Check sheet for the modelled part. Datum: model origin and axes. Units: mm. Face numbers are marked on the shaded views. A direction names the side the tool comes from. Round coordinates to 2 decimals unless told otherwise and drop trailing zeros. Loops run counter-clockwise (first coordinate to the right, second up) from the corner with the lowest first, then second, coordinate; pieces in that order, holes last. Notation, with made-up numbers: (78.5, -31) - (86.5, -31) arc R9 ccw to (86.5, -23) - close; hole circle Ø7 at (18.5, 58.5). An arc over 180 degrees is marked (long way). Put each result on its own line as item: value.
```python
from build123d import *

# Parameters (mm, degrees)
EXTRUDE_1_DEPTH = 6
EXTRUDE_2_DEPTH = 7
SKETCH_2_6_W    = 17.5
SKETCH_2_6_H    = 7
EXTRUDE_3_DEPTH = 28.5
CHAMFER_1_SIZE  = 4
HOLE_WIZARD_1_D = 8
FILLET_1_R      = 1
CHAMFER_2_SIZE  = 1


with BuildPart() as part:
    # Sketch 2 → Extrude 1 (new, symmetric)
    with BuildSketch(Plane.XY):
        with BuildLine():
            Line((-22.5, 0), (0, 0))
            Line((0, 0), (0, 20))
            Line((0, 20), (-10.5, 20))
            ThreePointArc((-10.5, 20), (-12, 21.5), (-10.5, 23))
            Line((-10.5, 23), (-10.5, 45))
            ThreePointArc((-10.5, 45), (-12, 46.5), (-10.5, 48))
            Line((-10.5, 48), (0, 48))
            Line((0, 48), (0, 55))
            Line((0, 55), (-22.5, 55))
            Line((-22.5, 55), (-22.5, 0))
        make_face()
        with BuildLine():
            Line((0, 20), (0, 0))
            Line((0, 0), (22.5, 0))
            Line((22.5, 0), (22.5, 55))
            Line((22.5, 55), (0, 55))
            Line((0, 55), (0, 48))
            Line((0, 48), (10.5, 48))
            ThreePointArc((10.5, 48), (11.560660172, 47.560660172), (12, 46.5))
            ThreePointArc((12, 46.5), (11.560660172, 45.439339828), (10.5, 45))
            Line((10.5, 45), (10.5, 23))
            ThreePointArc((10.5, 23), (11.560660172, 22.560660172), (12, 21.5))
            ThreePointArc((12, 21.5), (11.560660172, 20.439339828), (10.5, 20))
            Line((10.5, 20), (0, 20))
        make_face()
    extrude(amount=EXTRUDE_1_DEPTH, both=True)

    # Sketch 2_5 → Extrude 2 (add, symmetric)
    with BuildSketch(Plane.XY):
        Polygon((-22.5, 69), (-22.5, 55), (0, 55), (0, 62), (-17.5, 62), (-17.5, 69), align=None)
        Polygon((0, 55), (22.5, 55), (22.5, 69), (17.5, 69), (17.5, 62), (0, 62), align=None)
    extrude(amount=EXTRUDE_2_DEPTH, both=True)

    # Sketch 2_6 → Extrude 3 (add, symmetric)
    with BuildSketch(Plane.XY):
        with Locations((-8.75, 65.5)):
            Rectangle(SKETCH_2_6_W, SKETCH_2_6_H)
        with Locations((8.75, 65.5)):
            Rectangle(SKETCH_2_6_W, SKETCH_2_6_H)
        Polygon((0, 69), (17.5, 69), (17.5, 76), (10.5, 76), (10.5, 72), (0, 72), align=None)
        Polygon((-17.5, 76), (-17.5, 69), (0, 69), (0, 72), (-10.5, 72), (-10.5, 76), align=None)
    extrude(amount=EXTRUDE_3_DEPTH, both=True)

    # Chamfer 1
    chamfer_1_edges = [part.edges().sort_by_distance(p)[0] for p in [
        (17.5, 76, 0),
        (-17.5, 76, 0),
    ]]
    chamfer(chamfer_1_edges, length=CHAMFER_1_SIZE)

    # Hole Wizard 1 (through all)
    with Locations(Plane(origin=(0, 72, 0), x_dir=(1, 0, 0), z_dir=(0, 1, 0))):
        with Locations((0, 18.5), (0, -18.5)):
            Hole(HOLE_WIZARD_1_D / 2)

    # Fillet 1
    fillet_1_edges = [part.edges().sort_by_distance(p)[0] for p in [
        (17.5, 65.5, -7),
        (17.5, 69, 0),
        (0, 62, 7),
        (-17.5, 65.5, 7),
        (-17.5, 69, 0),
        (17.5, 65.5, 7),
        (-17.5, 65.5, -7),
        (0, 62, -7),
    ]]
    fillet(fillet_1_edges, radius=FILLET_1_R)

    # Chamfer 2
    chamfer_2_edges = [part.edges().sort_by_distance(p)[0] for p in [
        (22.5, 69, 0),
        (-22.5, 69, 0),
    ]]
    chamfer(chamfer_2_edges, length=CHAMFER_2_SIZE)


solid = part.part
```
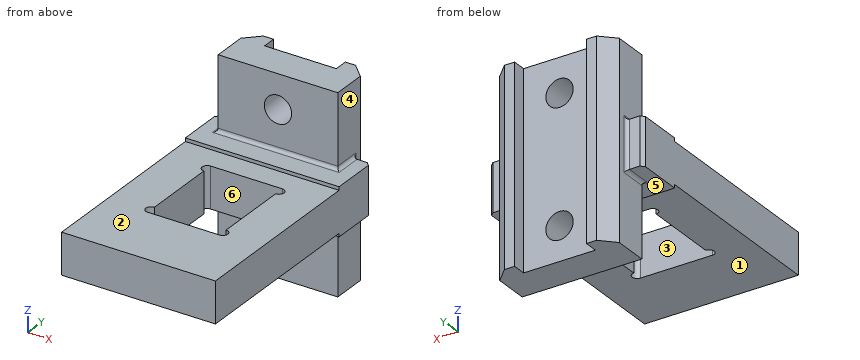
Item 1: Go/stop test with flat-tipped pins: pin 1 (1.5 mm diameter, centred on x = 4.5, z = -6, fed in from -Y); pin 2 (12 mm diameter, centred on x = 9.5, y = 35, fed in from +Z); pin 3 (12 mm diameter, centred on x = -3, z = 18.5, fed in from +Y); pin 4 (3 mm diameter, centred on y = 64.5, z = 11.5, fed in from +X). Record where each tip stops, or that it passes through.
Filled sheet:
pin 1: y = 0
pin 2: z = 6
pin 3: y = 72
pin 4: x = 17.5
Item 2: Release check for a two-part mould opening along X. For the marked faces 4, 5 and 6 record: +X half, -X half, draft (parallel to the pull), parting line (faces both ways), or undercut.
Filled sheet:
face 4: +X half
face 5: draft
face 6: undercut
Item 3: Tool access check on the marked faces 1, 2 and 3. Record the directions out of +Z, -Z, +X, -X, +Y, -Y that give a thin tool (end or side, any length) a straight path to the whole face; none if there is none.
Filled sheet:
face 1: -Z, +X, -X, -Y
face 2: +Z, +X, -X, -Y
face 3: +Z, -Z
Item 4: Section check B-B on z = 2. Enter the section's corners in (x, y).
Filled sheet:
outline: (-22.5, 0) - (22.5, 0) - (22.5, 68) - (21.5, 69) - (18.5, 69) arc R1 cw to (17.5, 70) - (17.5, 72) - (13.5, 76) - (10.5, 76) - (10.5, 72) - (-10.5, 72) - (-10.5, 76) - (-13.5, 76) - (-17.5, 72) - (-17.5, 70) arc R1 cw to (-18.5, 69) - (-21.5, 69) - (-22.5, 68) - close; hole (-10.5, 20) - (10.5, 20) arc R1.5 ccw to (10.5, 23) - (10.5, 45) arc R1.5 ccw to (10.5, 48) - (-10.5, 48) arc R1.5 ccw to (-10.5, 45) - (-10.5, 23) arc R1.5 ccw to start
Item 5: Section check D-D on x = 6. Enter the section's corners in (y, z), then the cut area to 3 significant figures.
Filled sheet:
outline: (0, -6) - (20, -6) - (20, 6) - (0, 6) - close; (48, -6) - (55, -6) - (55, -7) - (61, -7) arc R1 cw to (62, -8) - (62, -28.5) - (72, -28.5) - (72, 28.5) - (62, 28.5) - (62, 8) arc R1 cw to (61, 7) - (55, 7) - (55, 6) - (48, 6) - close
area: 992 mm²
Item 6: Section check C-C on y = 24. Enter the section's corners in (x, z).
Filled sheet:
outline: (-22.5, -6) - (-10.5, -6) - (-10.5, 6) - (-22.5, 6) - close; (10.5, -6) - (22.5, -6) - (22.5, 6) - (10.5, 6) - close
Item 7: Section check A-A on x = 0. Enter the section's corners in (y, z).
Filled sheet:
outline: (0, -6) - (20, -6) - (20, 6) - (0, 6) - close; (48, -6) - (55, -6) - (55, -7) - (61, -7) arc R1 cw to (62, -8) - (62, -14.5) - (72, -14.5) - (72, 14.5) - (62, 14.5) - (62, 8) arc R1 cw to (61, 7) - (55, 7) - (55, 6) - (48, 6) - close; (62, -28.5) - (72, -28.5) - (72, -22.5) - (62, -22.5) - close; (62, 22.5) - (72, 22.5) - (72, 28.5) - (62, 28.5) - close
Item 8: Thickness scan on line 1 (Z direction, x = 0, y = 66); line 2 (Y direction, x = -3, z = 4); line 3 (X direction, y = 21.5, z = 4.5). Record the ranges inside material, lowest first. Write a range as from..to.
Filled sheet:
line 1: -28.5..-22.5, -14.5..14.5, 22.5..28.5
line 2: 0..20, 48..72
line 3: -22.5..-12, 12..22.5
